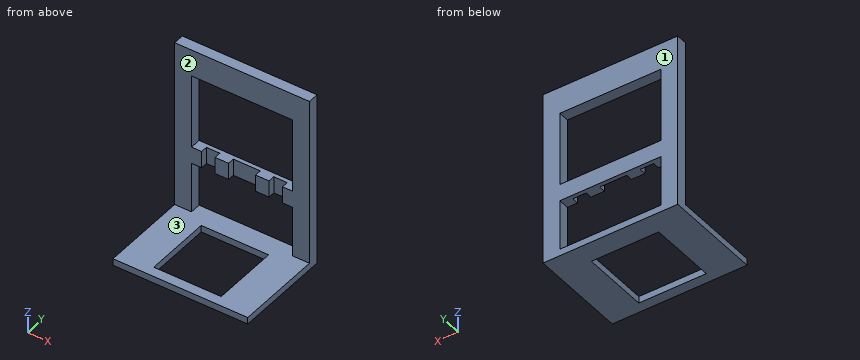
from build123d import *

# Parameters (mm, degrees)
SKETCH_3_W          = 10
SKETCH_3_H          = 1.5
EXTRUDE_1_DEPTH     = 1
EXTRUDE_2_DEPTH     = 1.6
CUT_EXTRUDE_1_REACH = 30.975
SKETCH_6_W          = 2
SKETCH_6_H          = 1
SKETCH_6_W_2        = 4


with BuildPart() as part:
    # 草图3 → 凸台-拉伸1 (new body)
    with BuildSketch(Plane.XY):
        Polygon((5, 7.602908894), (5, -2.397091106), (-5, -2.397091106), (-5, 7.602908894), (-5, 9.102908894), (-10, 9.102908894), (-10, -3.897091106), (10, -3.897091106), (10, 9.102908894), (5, 9.102908894), align=None)
        with Locations((0, 8.352908894)):
            Rectangle(SKETCH_3_W, SKETCH_3_H)
    extrude(amount=EXTRUDE_1_DEPTH)

    # 草图4 → 凸台-拉伸2 (add)
    with BuildSketch(Plane(origin=(0, 9.102908894, 0), x_dir=(1, 0, 0), z_dir=(0, 1, 0))):
        Polygon((10, -1), (10, 0), (0, 0), (0, -1), (7.5, -1), align=None)
        Polygon((0, -1), (0, 0), (-10, 0), (-10, -1), (-7.5, -1), align=None)
        Polygon((-7.5, -1), (-10, -1), (-10, -26), (0, -26), (0, -22), (-7.5, -22), (-7.5, -11), (0, -11), (0, -8.5), (-7.5, -8.5), align=None)
        Polygon((10, -26), (10, -1), (7.5, -1), (7.5, -8.5), (0, -8.5), (0, -11), (7.5, -11), (7.5, -22), (0, -22), (0, -26), align=None)
    extrude(amount=EXTRUDE_2_DEPTH)

    # 草图6 → 切除-拉伸1 (cut, up to next)
    with BuildSketch(Plane.XY.offset(1), mode=Mode.PRIVATE) as cut_extrude_1_sk1:
        with Locations((-5, 9.602908894)):
            Rectangle(SKETCH_6_W, SKETCH_6_H)
    cut_extrude_1_tool1 = extrude(cut_extrude_1_sk1.sketch, amount=CUT_EXTRUDE_1_REACH, mode=Mode.PRIVATE) & part.part
    # 草图6 → 切除-拉伸1 (cut, up to next)
    with BuildSketch(Plane.XY.offset(1), mode=Mode.PRIVATE) as cut_extrude_1_sk2:
        with Locations((5, 9.602908894)):
            Rectangle(SKETCH_6_W, SKETCH_6_H)
    cut_extrude_1_tool2 = extrude(cut_extrude_1_sk2.sketch, amount=CUT_EXTRUDE_1_REACH, mode=Mode.PRIVATE) & part.part
    # 草图6 → 切除-拉伸1 (cut, up to next)
    with BuildSketch(Plane.XY.offset(1), mode=Mode.PRIVATE) as cut_extrude_1_sk3:
        with Locations((0, 9.602908894)):
            Rectangle(SKETCH_6_W_2, SKETCH_6_H)
    cut_extrude_1_tool3 = extrude(cut_extrude_1_sk3.sketch, amount=CUT_EXTRUDE_1_REACH, mode=Mode.PRIVATE) & part.part
    add(cut_extrude_1_tool1.solids().sort_by_distance((-5, 9.602909, 1))[0], mode=Mode.SUBTRACT)
    add(cut_extrude_1_tool2.solids().sort_by_distance((5, 9.602909, 1))[0], mode=Mode.SUBTRACT)
    add(cut_extrude_1_tool3.solids().sort_by_distance((0, 9.602909, 1))[0], mode=Mode.SUBTRACT)


solid = part.part
For this review, take the finished solid that the model builds, in its own axes (mm). Face numbers are marked on the shaded views. A direction names the side the tool comes from. Coordinates: 2 decimals unless noted, no trailing zeros. Order: outer loops, then holes, each group sorted by start corner. A loop starts at its lowest first (then second) coordinate and runs counter-clockwise, first axis right, second up. Notation, with made-up numbers: (85, 0.5) - (107, 0.5) arc R28 cw to (107, 20.5) - close; hole circle Ø11 at (86.25, 62.25). An arc over 180 degrees is marked (long way). Use one line per item in the form item = value.
Q1. For the marked faces 1, 2 and 3, list the 3-axis set-ups (+Z, -Z, +X, -X, +Y, -Y) from which the entire face can be reached by the end or side of a thin tool; tool diameter is ignored.
Checked values:
face_1 = +Z, -Z, +X, -X, +Y
face_2 = +Z, +X, -X, -Y
face_3 = -Y
Q2. For P1, Ø1.6, axis at x = 5, z = 10, coming from the -Y side; P2, Ø2, axis at x = -5.5, z = 9, coming from the -Y side; P3, Ø4, axis at x = -7.5, y = -0.5, coming from the +Z side; P4, Ø0.5, axis at x = -3.5, y = 9.5, coming from the -Z side, all flat-tipped, find the tip position at first contact; note any pin that passes through.
Checked values:
P1 = 10.1
P2 = 9.1
P3 = 1
P4 = 0
Q3. Consider section C-C (y = 5). Give the boundary of the cut face in (x, z).
Checked values:
outline = (-10, 0) - (-5, 0) - (-5, 1) - (-10, 1) - close; (5, 0) - (10, 0) - (10, 1) - (5, 1) - close
Q4. Consider section B-B (z = 6.5). Give the boundary of the cut face in (x, y).
Checked values:
outline = (-10, 9.1) - (-7.5, 9.1) - (-7.5, 10.7) - (-10, 10.7) - close; (7.5, 9.1) - (10, 9.1) - (10, 10.7) - (7.5, 10.7) - close
Q5. Consider section D-D (x = 1.5). Give the boundary of the cut face in (y, z).
Checked values:
outline = (-3.9, 0) - (-2.4, 0) - (-2.4, 1) - (-3.9, 1) - close; (7.6, 0) - (10.7, 0) - (10.7, 1) - (7.6, 1) - close; (9.1, 22) - (10.7, 22) - (10.7, 26) - (9.1, 26) - close; (10.1, 8.5) - (10.7, 8.5) - (10.7, 11) - (10.1, 11) - close
Q6. For probe 1 along X at (y, z) = (9.25, 1.5); probe 2 along Y at (x, z) = (-1, 9); probe 3 along Z at (x, y) = (9, 3.25), list the stretches that pass through material, from the lowest coordinate up. Write a range as from..to.
Checked values:
probe_1 = -10..-7.5, 7.5..10
probe_2 = 10.1..10.7
probe_3 = 0..1
Q7. Consider section A-A (x = 6.5). Give the boundary of the cut face in (y, z).
Checked values:
outline = (-3.9, 0) - (10.7, 0) - (10.7, 1) - (-3.9, 1) - close; (9.1, 8.5) - (10.7, 8.5) - (10.7, 11) - (9.1, 11) - close; (9.1, 22) - (10.7, 22) - (10.7, 26) - (9.1, 26) - close
